Read the model definition and answer for the solid it produces. Units are mm, in the model's axes. Face numbers are marked on the shaded views. A direction names the side the tool comes from. Round coordinates to 2 decimals unless told otherwise and drop trailing zeros. Write each loop counter-clockwise with the first axis right and the second up, starting at its lowest first coordinate (ties: lowest second). Pieces come first, ordered by that corner, then holes. Notation, with made-up numbers: (30.25, 84) -> (39.25, 84) arc R15 ccw to (39.25, 89) -> close; hole circle Ø6 at (75.5, 55). An arc over 180 degrees is marked (long way). Return JSON: item names as keys, results as strings.
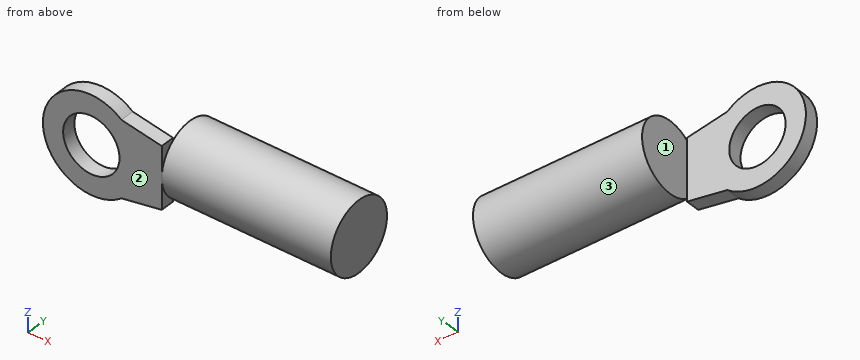
from build123d import *

# Parameters (mm, degrees)
SKETCH1_R           = 1.6
BOSS_EXTRUDE1_DEPTH = 0.8
SKETCH2_R           = 2
BOSS_EXTRUDE2_DEPTH = 9.6


with BuildPart() as part:
    # Sketch1 → Boss-Extrude1 (new body)
    with BuildSketch(Plane(origin=(0, 0, 0), x_dir=(1, 0, 0), z_dir=(0, 1, 0))):
        with BuildLine():
            Line((4, -1.75), (4, 1.75))
            Line((4, 1.75), (1.71464282, 2.15))
            ThreePointArc((1.71464282, 2.15), (-2.75, 0), (1.71464282, -2.15))
            Line((1.71464282, -2.15), (4, -1.75))
        make_face()
        Circle(SKETCH1_R, mode=Mode.SUBTRACT)
    extrude(amount=BOSS_EXTRUDE1_DEPTH)

    # Sketch2 → Boss-Extrude2 (add)
    with BuildSketch(Plane(origin=(4, 0, 0), x_dir=(0, 0, -1), z_dir=(1, 0, 0))):
        with Locations((0, 2)):
            Circle(SKETCH2_R)
    extrude(amount=BOSS_EXTRUDE2_DEPTH)


solid = part.part
Item 1: A tool of negligible diameter and unlimited length cuts with its end or side. For the marked faces 1, 2 and 3, from which of +Z, -Z, +X, -X, +Y, -Y can it reach the whole face along a straight path? Write none if from no direction.
Worked answers:
{"face 1": "+Z, -Z, -X, +Y", "face 2": "+Z, -Z, +X, -X, -Y", "face 3": "+X"}
Item 2: Section D-D (x = 4.25) is taken. Give the vertices of the cut face in (y, z), then the cut area to 3 significant figures.
Worked answers:
{"outline": "circle Ø4 at (2, 0)", "area": "12.6 mm2"}
Item 3: Section B-B (z = 1.4) is taken. Give the vertices of the cut face in (x, y), then the cut area to 3 significant figures.
Worked answers:
{"outline": "(-2.37, 0) -> (-0.77, 0) -> (-0.77, 0.8) -> (-2.37, 0.8) -> close; (0.77, 0) -> (4, 0) -> (4, 0.57) -> (13.6, 0.57) -> (13.6, 3.43) -> (4, 3.43) -> (4, 0.8) -> (0.77, 0.8) -> close", "area": "31.3 mm2"}
Item 4: Flat-ended cylindrical pins translate along their axes: pin 1 (1.6 mm diameter, centred on y = 1.5, z = -0.5, fed in from -X); pin 2 (1.7 mm diameter, centred on x = -1, z = -1.5, fed in from +Y). Find the tip coordinate at first contact, or state that the pin passes through.
Worked answers:
{"pin 1": "stops at x = -2.75", "pin 2": "stops at y = 0.8"}
Item 5: Section C-C (y = 0.6) is taken. Give the vertices of the cut face in (x, z).
Worked answers:
{"outline": "(1.71, -2.15) -> (4, -1.75) -> (4, -1.43) -> (13.6, -1.43) -> (13.6, 1.43) -> (4, 1.43) -> (4, 1.75) -> (1.71, 2.15) arc R2.75 ccw (long way) to start; hole circle Ø3.2 at (0, 0)"}
Item 6: Straight lines are drawn through the part: L1, parallel to Z at x = 0, y = 0.4; L2, parallel to X at y = 0.6, z = 0; L3, parallel to Y at x = 1.5, z = -1.5. For each, find the intervals that lie inside material, in ascending order. Write a range as [from, to].
Worked answers:
{"L1": "z = [-2.75, -1.6], [1.6, 2.75]", "L2": "x = [-2.75, -1.6], [1.6, 13.6]", "L3": "y = [0, 0.8]"}
Item 7: Section A-A (x = 0) is taken. Give the vertices of the cut face in (y, z), then the cut area to 3 significant figures.
Worked answers:
{"outline": "(0, -2.75) -> (0.8, -2.75) -> (0.8, -1.6) -> (0, -1.6) -> close; (0, 1.6) -> (0.8, 1.6) -> (0.8, 2.75) -> (0, 2.75) -> close", "area": "1.84 mm2"}
